Input: dimensioned drawing with shaded views. Units: mm. Origin: part minimum x, y, z. Round coordinates to 2 decimals unless told otherwise and drop trailing zeros. Loops run counter-clockwise (first coordinate to the right, second up) from the corner with the lowest first, then second, coordinate; pieces in that order, holes last. Notation, with made-up numbers: M 14,-30 L 44,-30 A15 cw 44,-20 Z; hole C 53.5,10.25 d5. An arc over 180 degrees is marked long. Write each question's results on one line, items separated by ' | '. Start each with the question number.
1. Draft query along Z for the marked faces 1, 2 and 3. Return one class per face: released by +Z, released by -Z, zero draft, split by the parting line, or undercut.
2. Contact query for flat-ended pins moving along their axis: pin 1 Ø4 at (x, y) = (13, 48.5) entering from +Z; pin 2 Ø10 at (x, y) = (41, 31.5) entering from -Z; pin 3 Ø12 at (x, y) = (43, 36.5) entering from -Z. Output: stop coordinate, or through.
3. Ray query, line 1 (X direction, y = 42, z = 25); line 2 (X direction, y = 31, z = 29.5). Return the intervals inside material, ascending.
4. Section A-A on x = 23. Output: boundary loops of the cut face in (y, z) (1 decimal).
5. Section B-B on z = 19. Output: boundary loops of the cut face in (x, y).
6. Section C-C on y = 51. Output: boundary loops of the cut face in (x, z) (1 decimal).
7. Section D-D on x = 6. Output: boundary loops of the cut face in (y, z).
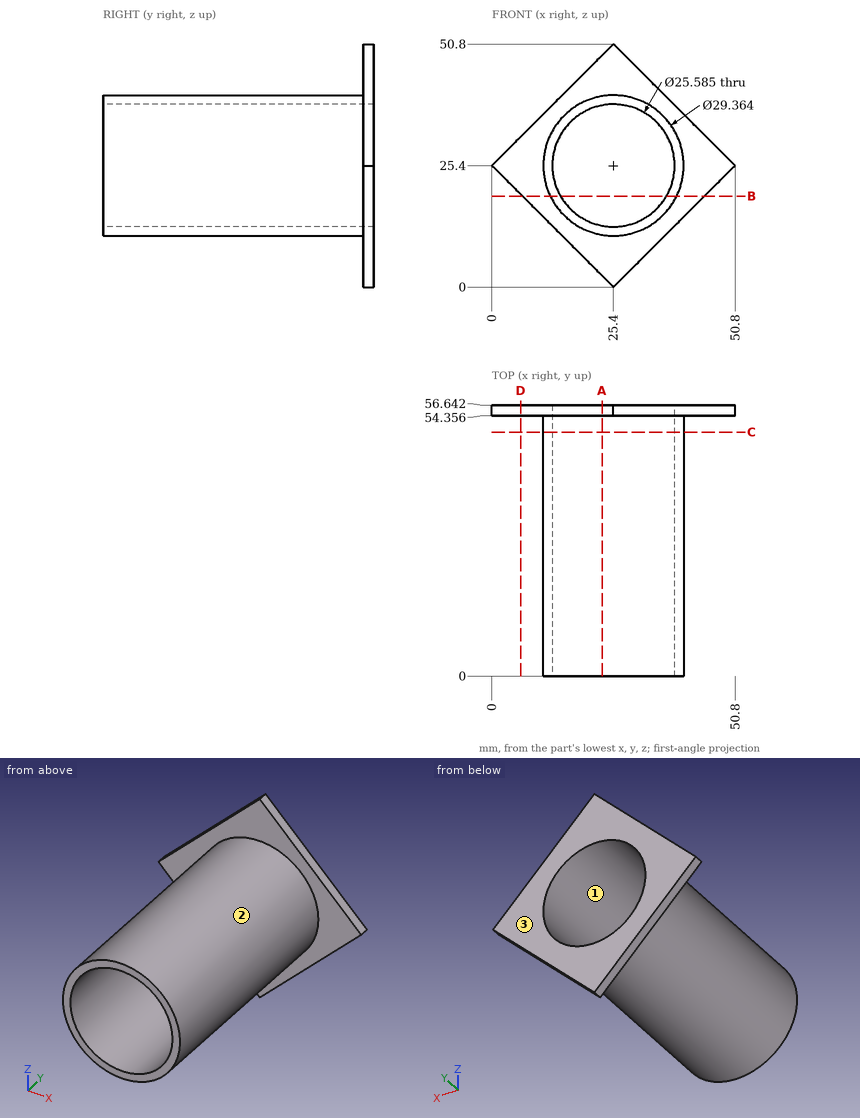
Taken from the geometry:
1) face 1: undercut | face 2: split by the parting line | face 3: zero draft
2) pin 1: z = 35.76 | pin 2: z = 15.24 | pin 3: z = 16.4
3) line 1: 10.72 to 12.61, 38.19 to 40.08 | line 2: 11.3 to 13.28, 37.52 to 39.5
4) outline: M 0,10.9 L 54.4,10.9 L 54.4,2.4 L 56.6,2.4 L 56.6,12.8 L 0,12.8 Z; M 0,38 L 56.6,38 L 56.6,48.4 L 54.4,48.4 L 54.4,39.9 L 0,39.9 Z
5) outline: M 6.4,54.36 L 12.19,54.36 L 12.19,0 L 14.32,0 L 14.32,56.64 L 6.4,56.64 Z; M 36.48,0 L 38.61,0 L 38.61,54.36 L 44.4,54.36 L 44.4,56.64 L 36.48,56.64 Z
6) outline: C 25.4,25.4 d29.4; hole C 25.4,25.4 d25.6
7) outline: M 54.36,19.4 L 56.64,19.4 L 56.64,31.4 L 54.36,31.4 Z
